Print and shaded views of the part. All mm, measured from the part's lowest x, y and z. A direction names the side the tool comes from. Round coordinates to 2 decimals unless told otherwise and drop trailing zeros. Loops run counter-clockwise (first coordinate to the right, second up) from the corner with the lowest first, then second, coordinate; pieces in that order, holes last. Notation, with made-up numbers: (33.25, 22.5) - (85.25, 22.5) arc R26 ccw to (85.25, 41.5) - close; hole circle Ø6 at (58.25, 77.5). An arc over 180 degrees is marked (long way). Answer as a JSON object with one key per item and string values.
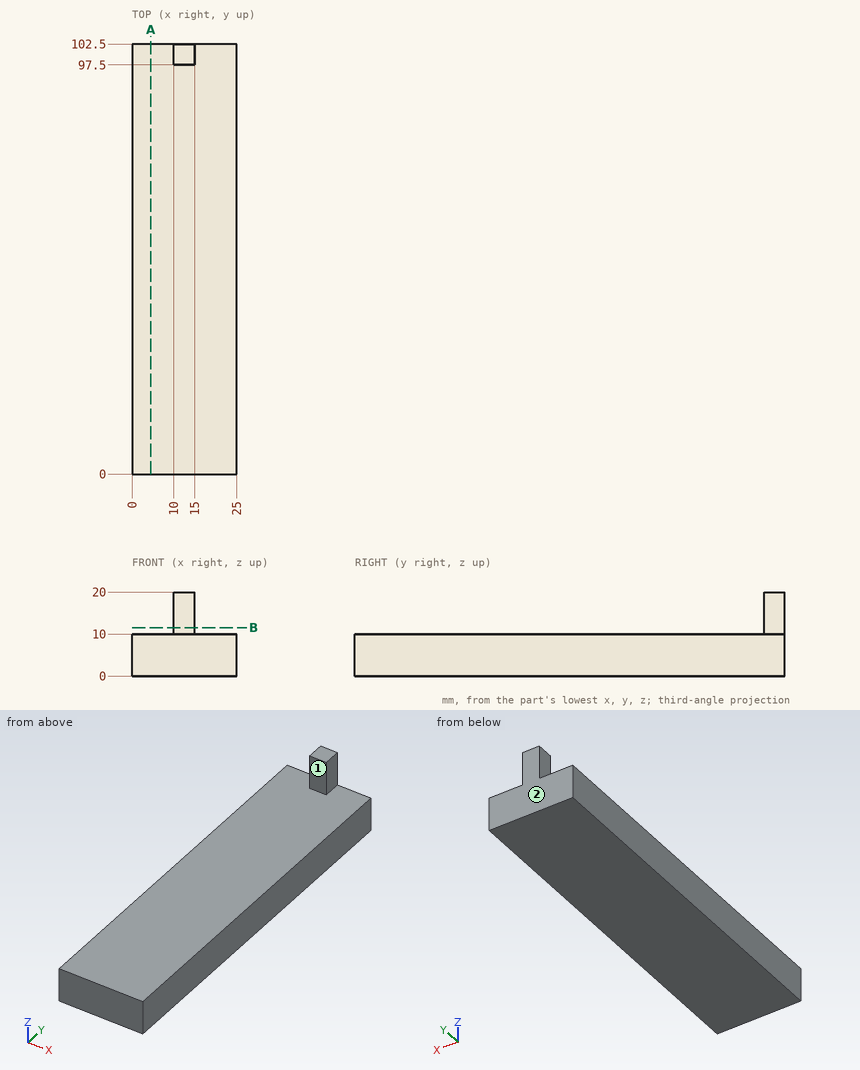
1) Slice it at B-B on z = 11.5. List the corners of the cut face in (x, y), then the cut area to 3 significant figures.
Values follow:
{"outline": "(10, 97.5) - (15, 97.5) - (15, 102.5) - (10, 102.5) - close", "area": "25.0 mm²"}
2) Slice it at A-A on x = 4.5. List the corners of the cut face in (y, z), then the cut area to 4 significant figures.
Values follow:
{"outline": "(0, 0) - (102.5, 0) - (102.5, 10) - (0, 10) - close", "area": "1,025 mm²"}
3) Drop flat-ended pins along their axis: P1, Ø7.5, axis at x = 13.5, y = 50, coming from the +Z side; P2, Ø4, axis at y = 100.5, z = 13, coming from the -X side; P3, Ø5.5, axis at y = 101, z = 14.5, coming from the +X side. Give the stop position or say it passes through.
Values follow:
{"P1": "z = 10", "P2": "x = 10", "P3": "x = 15"}
4) Tool access for the marked faces 1 and 2: list every direction of +Z, -Z, +X, -X, +Y, -Y with a clear straight run to the whole face (end or side of a thin tool).
Values follow:
{"face 1": "+Z, +X, -X, -Y", "face 2": "+Z, -Z, +X, -X, +Y"}
5) Probe probe 1 along Z at (x, y) = (19.5, 71.5); probe 2 along Y at (x, z) = (14.5, 17.25). List the from-to ranges inside material, lowest first.
Values follow:
{"probe 1": "0 to 10", "probe 2": "97.5 to 102.5"}
